Could you check a few things on this model? Use its own coordinates, in mm. Give positions to 0.01 mm unless a question says otherwise; leave off trailing zeros. Loops run counter-clockwise (first coordinate to the right, second up) from the corner with the lowest first, then second, coordinate; pieces in that order, holes last. Notation, with made-up numbers: (73, 4) -> (82, 4) arc R29 ccw to (82, 37) -> close; hole circle Ø9 at (23.5, 48.25). An arc over 180 degrees is marked (long way). Put each result on its own line as item: value.
```python
from build123d import *

# Parameters (mm, degrees)
F1_DEPTH = 13


with BuildPart() as f1:
    # F0 (on Front) → F1 (new body)
    with BuildSketch(Plane.XZ):
        with BuildLine():
            Line((0, 35.834754), (0, -22.5))
            ThreePointArc((0, -22.5), (15.909903, -15.909903), (22.5, 0))
            ThreePointArc((22.5, 0), (19.52034, 16.102515), (10.975956, 30.072585))
            ThreePointArc((10.975956, 30.072585), (9.319805, 31.819805), (7.572585, 33.475956))
            ThreePointArc((7.572585, 33.475956), (3.965727, 35.231404), (0, 35.834754))
        make_face()
        with BuildLine():
            ThreePointArc((7.572585, 33.475956), (9.319805, 31.819805), (10.975956, 30.072585))
            ThreePointArc((10.975956, 30.072585), (9.429095, 31.929095), (7.572585, 33.475956))
        make_face()
    extrude(amount=F1_DEPTH)


solid = f1.part
```
1. If we section it at C-C (x = 13.5): List the corners of the cut face in (y, z) for me, then the cut area to 3 significant figures.
Recorded:
outline: (-13, -18) -> (0, -18) -> (0, 27) -> (-13, 27) -> close
area: 585 mm^2
2. If we section it at A-A (y = -1.25): List the corners of the cut face in (x, z) for me.
Recorded:
outline: (0, -22.5) arc R22.5 ccw to (22.5, 0) arc R45 ccw to (10.98, 30.07) arc R13.33 ccw to (7.57, 33.48) arc R13.33 ccw to (0, 35.83) -> close
3. Thinking about a two-plate mould opening in X: for faces 1 (the face through (19.6, -6.41, 15.89)), 2 (the face through (0, -6, 7)), 3 (the face through (9, 0, 7)), which applies, pulls with the +X half, pulls with the -X half, needs draft (parallel to the pull), parting line crosses it, or undercut?
Recorded:
face 1: pulls with the +X half
face 2: pulls with the -X half
face 3: needs draft
4. I'm going to push flat-ended pins straight in: pin 1 (1 mm diameter, centred on y = -6, z = 6, fed in from +X); pin 2 (1.5 mm diameter, centred on x = 4, y = -8.5, fed in from -Z). Where does each tip first touch, or does it pass through?
Recorded:
pin 1: stops at x = 22.16
pin 2: stops at z = -22.26
5. I need wall thicknesses on line 1 (X direction, y = -1.25, z = -6); line 2 (Z direction, x = 1, y = -8.75); line 3 (Z direction, x = 10.75, y = -11.5). Which ranges of each line are inside material? Lowest first, please.
Recorded:
line 1: x = 0 to 21.69
line 2: z = -22.48 to 35.8
line 3: z = -19.77 to 30.39
6. If we section it at B-B (z = 27): List the corners of the cut face in (x, y) for me.
Recorded:
outline: (0, -13) -> (13.5, -13) -> (13.5, 0) -> (0, 0) -> close
